Verification items for the finished model (mm, model axes). Round coordinates to 2 decimals unless told otherwise and drop trailing zeros. Write each loop counter-clockwise with the first axis right and the second up, starting at its lowest first coordinate (ties: lowest second). Pieces come first, ordered by that corner, then holes. Notation, with made-up numbers: (-25, 14.25) - (6, 14.25) arc R17 ccw to (6, 25.25) - close; hole circle Ø2 at (46.25, 78.5). An arc over 180 degrees is marked (long way). Answer as a JSON object with one key per item and string values. Group by question number.
1) Section check C-C (y = 6.5). Enter the section's corners in (x, z) (1 decimal).
2) Mould release check, pull along Z, two halves, no side actions. Record for faces 1 (the cylindrical face through (3.78, 4.7, 2.9)), 2 (the cylindrical face through (14.274, 4.705, -0.628)), 3 (the flat face through (0, 0, -6)): +Z half, -Z half, draft (parallel to the pull), parting line (faces both ways), or undercut.
3) Section check A-A (x = 0). Enter the section's corners in (y, z) (1 decimal), then the cut area to 3 significant figures.
4) Section check B-B (z = 0). Enter the section's corners in (x, y) (1 decimal).
5) Go/stop test with a flat-tipped pin: pin 1 Ø3 at (x, y) = (-10.5, 1) entering from +Z. Record where the tip stops, or that it passes through.
6) Thickness scan on line 1 (Z direction, x = 0, y = 5.25); line 2 (X direction, y = 5.5, z = -4); line 3 (Z direction, x = -3.5, y = 1.5). Record the ranges inside material, lowest first.
Autodesk Inventor part; units mm, degrees
ref_plane "YZ Plane" through (0, 0, 0) normal (1, 0, 0) x (0, 1, 0)
ref_plane "XZ Plane" through (0, 0, 0) normal (0, 1, 0) x (-1, 0, 0)
ref_plane "XY Plane" through (0, 0, 0) normal (0, 0, 1) x (1, 0, 0)
sketch "Sketch1" plane through (0, 0, 0) normal (0, 1, 0) x (-1, 0, 0)
  circle A0 centre (0, 0) radius 4.7625
  circle A1 centre (0, 0) radius 14.2875
  dimension "d0" = 9.525
  dimension "d1" = 28.575
extrude "Extrusion1" add sketch "Sketch1" along normal blind 9.525
fillet "Fillet1" radius 0.635 1 edges at (14.2875, 9.525, 0)
fillet "Fillet2" radius 0.635 1 edges at (14.2875, 0, 0)
fillet "Fillet3" radius 0.635 1 edges at (4.7625, 9.525, 0)
fillet "Fillet4" radius 0.635 1 edges at (4.7625, 0, 0)
properties part number "1614zz bearing"
Returned:
{
 "1": {"outline": "circle Ø28.6 at (0, 0); hole circle Ø9.5 at (0, 0)"},
 "2": {"face 1": "undercut", "face 2": "parting line", "face 3": "draft"},
 "3": {"outline": "(0, -13.7) arc R0.6 ccw to (0.6, -14.3) - (8.9, -14.3) arc R0.6 ccw to (9.5, -13.7) - (9.5, -5.4) arc R0.6 ccw to (8.9, -4.8) - (0.6, -4.8) arc R0.6 ccw to (0, -5.4) - close; (0, 5.4) arc R0.6 ccw to (0.6, 4.8) - (8.9, 4.8) arc R0.6 ccw to (9.5, 5.4) - (9.5, 13.7) arc R0.6 ccw to (8.9, 14.3) - (0.6, 14.3) arc R0.6 ccw to (0, 13.7) - close", "area": "181 mm2"},
 "4": {"outline": "(-14.3, 0.6) arc R0.6 ccw to (-13.7, 0) - (-5.4, 0) arc R0.6 ccw to (-4.8, 0.6) - (-4.8, 8.9) arc R0.6 ccw to (-5.4, 9.5) - (-13.7, 9.5) arc R0.6 ccw to (-14.3, 8.9) - close; (4.8, 0.6) arc R0.6 ccw to (5.4, 0) - (13.7, 0) arc R0.6 ccw to (14.3, 0.6) - (14.3, 8.9) arc R0.6 ccw to (13.7, 9.5) - (5.4, 9.5) arc R0.6 ccw to (4.8, 8.9) - close"},
 "5": {"pin 1": "z = 11.1"},
 "6": {"line 1": "-14.29 to -4.76, 4.76 to 14.29", "line 2": "-13.72 to -2.58, 2.58 to 13.72", "line 3": "-13.85 to -3.23, 3.23 to 13.85"}
}
